Verification items for the finished model (mm, model axes). Round coordinates to 2 decimals unless told otherwise and drop trailing zeros. Write each loop counter-clockwise with the first axis right and the second up, starting at its lowest first coordinate (ties: lowest second). Pieces come first, ordered by that corner, then holes. Notation, with made-up numbers: M -29,-38.75 L 26,-38.75 A23 cw 26,-30.75 Z; hole C -13.5,25 d7. An arc over 180 degrees is marked long. Write each question's results on one line, items separated by ' | '.
from build123d import *

# Parameters (mm, degrees)
BOSS_EXTRUDE1_DEPTH = 35
SKETCH2_R           = 20
CUT_EXTRUDE1_DEPTH  = 36


with BuildPart() as part:
    # Sketch1 → Boss-Extrude1 (new body)
    with BuildSketch(Plane(origin=(0, 0, 0), x_dir=(1, 0, 0), z_dir=(0, 1, 0))):
        Polygon((30, 10), (10, 30), (-10, 30), (-30, 10), (-30, -10), (-10, -30), (10, -30), (30, -10), align=None)
    extrude(amount=BOSS_EXTRUDE1_DEPTH)

    # Sketch2 → Cut-Extrude1 (cut, through all)
    with BuildSketch(Plane(origin=(0, 35, 0), x_dir=(1, 0, 0), z_dir=(0, 1, 0))):
        Circle(SKETCH2_R)
    extrude(amount=-CUT_EXTRUDE1_DEPTH, mode=Mode.SUBTRACT)


solid = part.part
1) Draft check along Z on faces 1 (the cylindrical face through (-4.336, 17.745, 19.524)), 2 (the flat face through (-20, 17, -20)), 3 (the flat face through (20, 0, 6)). Enter one of: pulls with the +Z half, pulls with the -Z half, needs draft (parallel to the pull), parting line crosses it, or undercut.
Calculated:
face 1: undercut | face 2: pulls with the -Z half | face 3: needs draft
2) Depth check by flat-ended pin: P1, Ø5, axis at y = 10, z = 18, coming from the +X side; P2, Ø3, axis at y = 22, z = -23.5, coming from the +X side; P3, Ø10, axis at x = -18.5, y = 21, coming from the +Z side. Enter the tip coordinate at first touch or a pass-through.
Calculated:
P1: stops at x = 24.5 | P2: stops at x = 18 | P3: stops at z = 26.5
3) Sectioned sample at A-A, the plane x = 0. Record the cut outline in (y, z), and give its area (3 significant figures).
Calculated:
outline: M 0,-30 L 35,-30 L 35,-20 L 0,-20 Z; M 0,20 L 35,20 L 35,30 L 0,30 Z | area: 700 mm²
4) Sectioned sample at C-C, the plane y = 10. Record the cut outline in (x, z), and give its area (3 significant figures).
Calculated:
outline: M -30,-10 L -10,-30 L 10,-30 L 30,-10 L 30,10 L 10,30 L -10,30 L -30,10 Z; hole C 0,0 d40 | area: 1,540 mm²
5) Material ranges on line 1 (X direction, y = 11.5, z = 0); line 2 (Z direction, x = -5.5, y = 14), recorded low to high. Write a range as [from, to].
Calculated:
line 1: x = [-30, -20], [20, 30] | line 2: z = [-30, -19.23], [19.23, 30]
6) Sectioned sample at B-B, the plane z = 0. Record the cut outline in (x, y).
Calculated:
outline: M -30,0 L -20,0 L -20,35 L -30,35 Z; M 20,0 L 30,0 L 30,35 L 20,35 Z
